The listing builds one solid part. Answer for the finished solid, in the listing's coordinates (mm). A direction names the side the tool comes from. Round coordinates to 2 decimals unless told otherwise and drop trailing zeros. Order: outer loops, then holes, each group sorted by start corner. A loop starts at its lowest first (then second) coordinate and runs counter-clockwise, first axis right, second up. Notation, with made-up numbers: (13.25, 61.5) - (55.25, 61.5) arc R10 cw to (55.25, 76.5) - close; hole circle Ø10 at (65, -4.75). An arc over 180 degrees is marked (long way). Write item = value, one per line.
from build123d import *

# Parameters (mm, degrees)
F0_W     = 25.4
F0_H     = 76.2
F1_DEPTH = 12.7
F3_D     = 6.35
F5_DEPTH = 5.08
F6_R     = 5.08


with BuildPart() as f1:
    # F0 (on Top) → F1 (new body)
    with BuildSketch(Plane.XY):
        with Locations((12.7, -20.335565)):
            Rectangle(F0_W, F0_H)
    extrude(amount=F1_DEPTH)

    # F3 (through all)
    with Locations(Plane.XY.offset(12.7)):
        with Locations((17.470095, 5.998946)):
            Hole(F3_D / 2)

    # F4 (on Front) → F5 (join)
    with BuildSketch(Plane.XZ):
        with BuildLine():
            Line((13.889657, 0), (9.24853, 0))
            Line((9.24853, 0), (4.607402, 0))
            ThreePointArc((4.607402, 0), (3.231891, -4.050694), (4.607402, -8.101388))
            ThreePointArc((4.607402, -8.101388), (5.886924, -8.185929), (6.245447, -6.954757))
            ThreePointArc((6.245447, -6.954757), (5.325208, -5.387091), (5.299789, -3.569464))
            ThreePointArc((5.299789, -3.569464), (5.695978, -2.181126), (6.900665, -1.385403))
            ThreePointArc((6.900665, -1.385403), (8.074597, -1.140454), (9.24853, -1.385403))
            ThreePointArc((9.24853, -1.385403), (10.422462, -1.140454), (11.596394, -1.385403))
            ThreePointArc((11.596394, -1.385403), (12.801081, -2.181126), (13.19727, -3.569464))
            ThreePointArc((13.19727, -3.569464), (13.171851, -5.387091), (12.251612, -6.954757))
            ThreePointArc((12.251612, -6.954757), (12.610135, -8.185929), (13.889657, -8.101388))
            ThreePointArc((13.889657, -8.101388), (15.265168, -4.050694), (13.889657, 0))
        make_face()
    extrude(amount=F5_DEPTH)

    # F6
    f6_edges = [f1.edges().sort_by_distance(p)[0] for p in [
        (0, 17.764435, 6.35),
        (25.4, 17.764435, 6.35),
        (12.7, 17.764435, 0),
    ]]
    fillet(f6_edges, radius=F6_R)


solid = f1.part
Q1. Section B-B on x = 16.5 is taken. Determine the outline of the cut face in (y, z), then the cut area to 3 significant figures.
Model answer:
outline = (-58.44, 0) - (2.98, 0) - (2.98, 12.7) - (-58.44, 12.7) - close; (9.02, 0) - (12.68, 0) arc R5.08 ccw to (17.76, 5.08) - (17.76, 12.7) - (9.02, 12.7) - close
area = 885 mm^2
Q2. Determine the mould class of faces 1 (the face through (9, 0, -1)), 2 (the face through (5.33, -2.5, -5.41)), 3 (the face through (25.4, -23, 6)) for opening direction X: released by +X, released by -X, zero draft, split by the parting line, or undercut.
Model answer:
face_1 = zero draft
face_2 = undercut
face_3 = released by +X
Q3. Section D-D on z = 9.5 is taken. Determine the outline of the cut face in (x, y) (3 decimals).
Model answer:
outline = (0, -58.436) - (25.4, -58.436) - (25.4, 12.684) arc R5.08 ccw to (20.32, 17.764) - (5.08, 17.764) arc R5.08 ccw to (0, 12.684) - close; hole circle Ø6.35 at (17.47, 5.999)
Q4. Section A-A on z = -2.5 is taken. Determine the outline of the cut face in (x, y), then the cut area to 3 significant figures.
Model answer:
outline = (3.42, -5.08) - (5.5, -5.08) - (5.5, 0) - (3.42, 0) - close; (12.99, -5.08) - (15.08, -5.08) - (15.08, 0) - (12.99, 0) - close
area = 21.2 mm^2
Q5. Section C-C on y = 7 is taken. Determine the outline of the cut face in (x, z), then the cut area to 3 significant figures.
Model answer:
outline = (0, 0) - (14.46, 0) - (14.46, 12.7) - (0, 12.7) - close; (20.48, 0) - (25.4, 0) - (25.4, 12.7) - (20.48, 12.7) - close
area = 246 mm^2
Q6. Flat-ended cylindrical pins translate along their axes: P1, Ø12, axis at y = -31, z = -2, coming from the -X side; P2, Ø9, axis at x = 12, z = -5.5, coming from the -Y side; P3, Ø12.5, axis at x = 10, y = -24.5, coming from the -Z side. Find the tip coordinate at first contact, or state that the pin passes through.
Model answer:
P1 = 0
P2 = -5.08
P3 = 0
Q7. Find the intervals of material crossed by line 1 (Z direction, x = 15.25, y = 3); line 2 (Y direction, x = 18.75, z = 10.75); line 3 (Y direction, x = 14.75, z = -4), in increasing order. Write a range as from..to.
Model answer:
line_1 = 0..12.7
line_2 = -58.44..3.09, 8.9..17.76
line_3 = -5.08..0
Q8. For faces 4 (the face through (20.64, 6.14, 6.26)), 5 (the face through (5.68, -2.5, -2.2)), 6 (the face through (9, -5.08, -1)), determine the directions among +Z, -Z, +X, -X, +Y, -Y from which every point of the face is accessible in a straight line to the end or side of a thin tool.
Model answer:
face_4 = +Z, -Z
face_5 = +Y, -Y
face_6 = -Z, +X, -X, -Y
